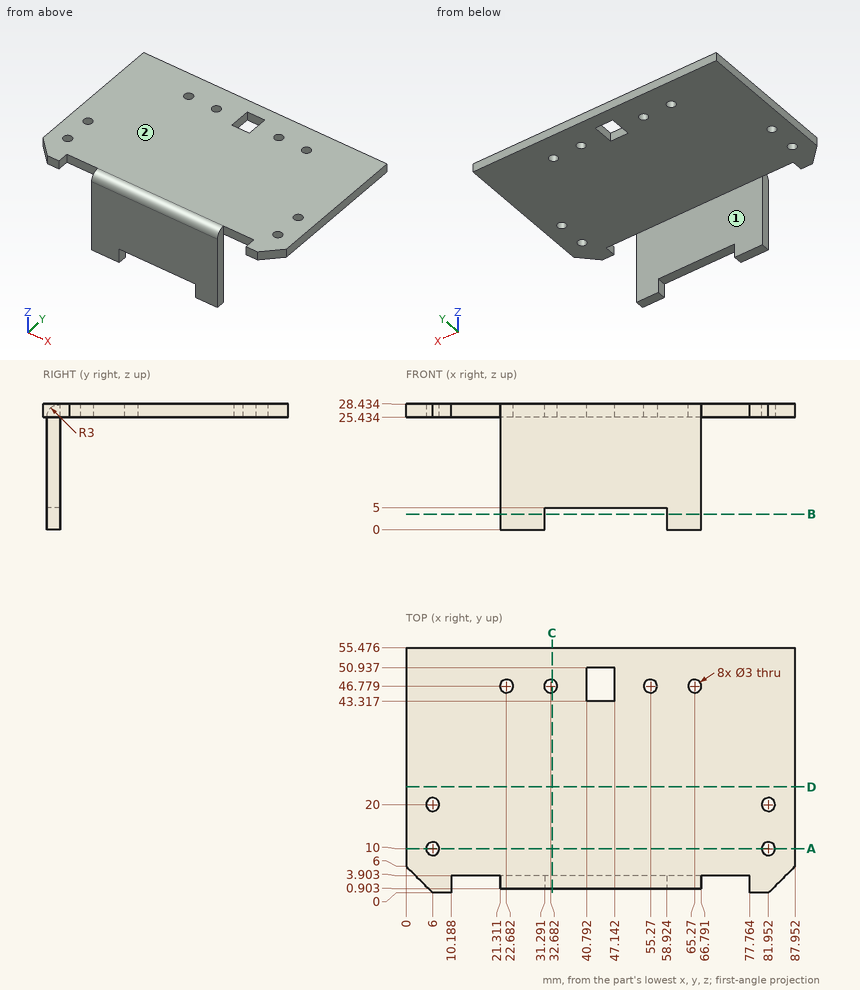
Drawing for the job (mm, zero at the part's lowest x, y, z). A direction names the side the tool comes from. Give positions to 0.01 mm unless a question says otherwise; leave off trailing zeros. Order: outer loops, then holes, each group sorted by start corner. A loop starts at its lowest first (then second) coordinate and runs counter-clockwise, first axis right, second up. Notation, with made-up numbers: M 48.5,-6 L 69.5,-6 A12 cw 69.5,2 Z; hole C 42.25,7 d6. An arc over 180 degrees is marked long. Use a Markdown table: item, result. Add a question column.
(1) Saw through at C-C, the plane x = 33. Give the cut face in (y, z) (1 decimal).
(2) 3-axis set-ups, long thin cutter, end or side, ignore diameter. For the marked faces 1 and 2: which of +Z, -Z, +X, -X, +Y, -Y reach the whole face in a straight line?
(3) Saw through at A-A, the plane y = 10. Give the cut face in (x, z) (1 decimal).
(4) Saw through at D-D, the plane y = 24. Give the cut face in (x, z) (1 decimal), and give its area (3 significant figures).
(5) Drop flat-ended pins along their axis: P1, Ø1.5, axis at y = 1, z = 27.5, coming from the -X side; P2, Ø0.9, axis at y = 3, z = 12.5, coming from the -X side; P3, Ø6, axis at x = 43, z = 3, coming from the -Y side; P4, Ø2.5, axis at x = 6, y = 20, coming from the +Z side. Give the stop position or say it passes through.
(6) Probe line 1 along Y through (x, z) = (6, 26.8) (1 decimal); line 2 along Y through (x, z) = (29, 19); line 3 along Z through (x, y) = (34, 12) (1 decimal). List the from-to ranges inside material, lowest first. Write a range as [from, to].
(7) Saw through at B-B, the plane z = 3.5. Give the cut face in (x, y).
Answer key:
| question | item | result |
|---|---|---|
| 1 | outline | M 0.9,5 L 3.9,5 L 3.9,25.4 L 45.3,25.4 L 45.3,28.4 L 3.9,28.4 A3 ccw 0.9,25.4 Z; M 48.2,25.4 L 55.5,25.4 L 55.5,28.4 L 48.2,28.4 Z |
| 2 | face 1 | -Z, +X, -X, +Y |
| 2 | face 2 | +Z, +X, -X, +Y, -Y |
| 3 | outline | M 0,25.4 L 4.5,25.4 L 4.5,28.4 L 0,28.4 Z; M 7.5,25.4 L 80.5,25.4 L 80.5,28.4 L 7.5,28.4 Z; M 83.5,25.4 L 88,25.4 L 88,28.4 L 83.5,28.4 Z |
| 4 | outline | M 0,25.4 L 88,25.4 L 88,28.4 L 0,28.4 Z |
| 4 | area | 264 mm^2 |
| 5 | P1 | x = 4.25 |
| 5 | P2 | x = 21.31 |
| 5 | P3 | y = 0.9 |
| 5 | P4 | through |
| 6 | line 1 | [0, 8.5], [11.5, 18.5], [21.5, 55.5] |
| 6 | line 2 | [0.9, 3.9] |
| 6 | line 3 | [25.4, 28.4] |
| 7 | outline | M 21.31,0.9 L 31.29,0.9 L 31.29,3.9 L 21.31,3.9 Z; M 58.92,0.9 L 66.79,0.9 L 66.79,3.9 L 58.92,3.9 Z |
